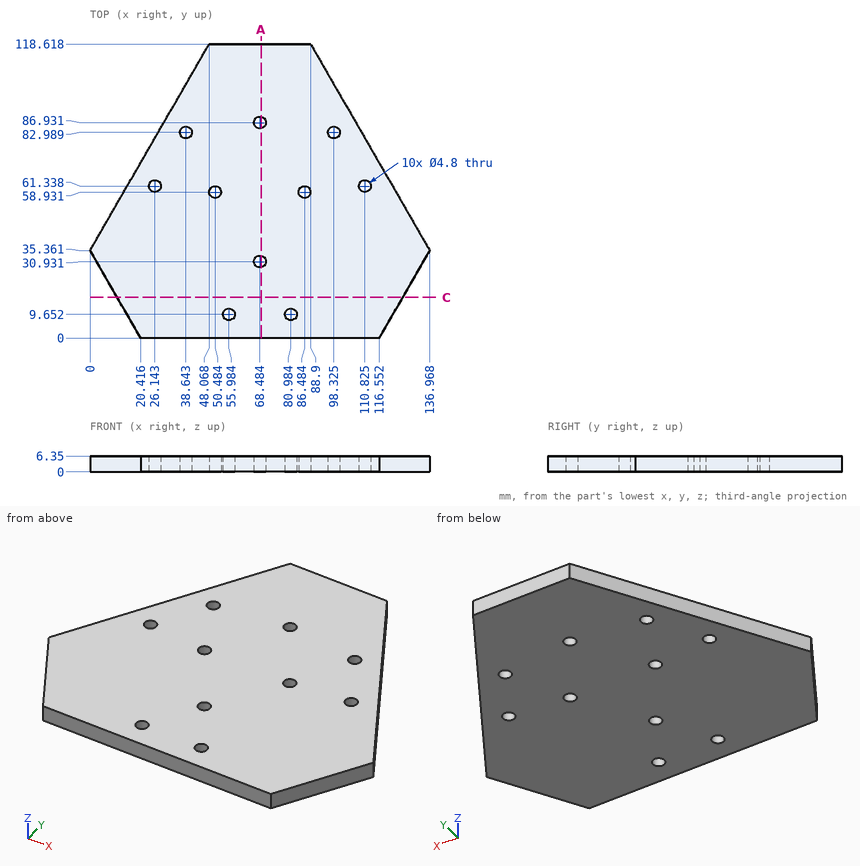
Design review of the part shown in the three views and the two pictorial views. Dimensions are in mm from the part's minimum x, y and z. Give positions to 0.01 mm unless a question says otherwise; leave off trailing zeros. Order: outer loops, then holes, each group sorted by start corner. A loop starts at its lowest first (then second) coordinate and runs counter-clockwise, first axis right, second up. Notation, with made-up numbers: (-17.75, -4.75) -> (39.25, -4.75) arc R20 cw to (39.25, 23.25) -> close; hole circle Ø5 at (-12.5, 38.5). An arc over 180 degrees is marked (long way). Write each question's results on one line, items separated by ' | '. Start each with the question number.
Q1. For pin 1 (1.5 mm diameter, centred on y = 51, z = 2, fed in from +X); pin 2 (1 mm diameter, centred on x = 17.5, z = 5.5, fed in from -Y) (1 decimal); pin 3 (1 mm diameter, centred on y = 92, z = 5.5, fed in from -X), all flat-tipped, find the tip position at first contact; note any pin that passes through.
Q2. Wall thickness on L1, parallel to X at y = 11, z = 2.5 (1 decimal); L2, parallel to Y at x = 54, z = 6.25 (1 decimal); L3, parallel to X at y = 31.5, z = 0.5 (1 decimal): over which ranges is each line inside the solid? List them lowest first. Write a range as from..to.
Q3. Add section C-C on y = 16.5. Give the boundary of the cut face in (x, z).
Q4. Add section A-A on x = 69. State how many separate pieces and enclosed holes the cut face has.
Found:
1) pin 1: stops at x = 128.37 | pin 2: stops at y = 4.2 | pin 3: stops at x = 32.41
2) L1: x = 14.1..54, 58..79, 83..122.9 | L2: y = 0..8.3, 11..118.6 | L3: x = 2.2..66.2, 70.8..134.7
3) outline: (10.89, 0) -> (126.08, 0) -> (126.08, 6.35) -> (10.89, 6.35) -> close
4) separate pieces: 3 | enclosed holes: 0
